Could you check a few things on this model? Use its own coordinates, in mm. Face numbers are marked on the shaded views. A direction names the side the tool comes from. Give positions to 0.01 mm unless a question says otherwise; leave off trailing zeros. Order: outer loops, then holes, each group sorted by start corner. A loop starts at its lowest first (then second) coordinate and runs counter-clockwise, first axis right, second up. Notation, with made-up numbers: (-3.75, -36) - (30.25, -36) arc R11 ccw to (30.25, -18) - close; hole circle Ø4 at (70.5, 18.25). An arc over 180 degrees is marked (long way). Put each result on its own line as item: value.
Autodesk Inventor part; units mm, degrees
ref_plane "YZ Plane" through (0, 0, 0) normal (1, 0, 0) x (0, 1, 0)
ref_plane "XZ Plane" through (0, 0, 0) normal (0, 1, 0) x (-1, 0, 0)
ref_plane "XY Plane" through (0, 0, 0) normal (0, 0, 1) x (1, 0, 0)
sketch "Sketch1" plane through (0, 0, 0) normal (0, 1, 0) x (-1, 0, 0)
  line L0 (-15, 15) -> (15, 15)
  line L1 (15, 15) -> (15, -15)
  line L2 (15, -15) -> (-15, -15)
  line L3 (-15, -15) -> (-15, 15)
  line L4 (-15, 15) -> (15, -15) construction
  line L5 (15, 15) -> (-15, -15) construction
  line L6 (-15, -15) -> (-15, -25)
  line L7 (-15, -25) -> (15, -15)
  point P0 (0, 0)
  dimension "d0" = 30
  dimension "d1" = 30
  dimension "d2" = 10
extrude "Extrusion1" add sketch "Sketch1" along normal blind 5
sketch "Sketch2" plane through (0, 5, 0) normal (0, 1, 0) x (1, 0, 0)
  line L0 (15, 25) -> (-15, 15)
  line L1 (15, 25) -> (18.0837, 15.7488)
  line L2 (15, -15) -> (15, 25)
  line L3 (15, 25) -> (6.9886, 22.3295)
  line L4 (-15, 15) -> (-9.6166, 16.7945)
  line L5 (-15, 15) -> (-13.1902, 9.5707)
  point P0 (0, 0)
ref_plane "Work Plane2" through (-15, 5, -15) normal (-0.9487, 0, 0.3162) x (0, -1, 0)
sketch "Sketch3" plane through (-15, 5, -15) normal (-0.9487, 0, 0.3162) x (0, -1, 0)
  line L0 (0, 37.9473) -> (0, 0)
  line L1 (0, 0) -> (-5, 0)
  line L2 (-5, 0) -> (-5, 3)
  line L3 (-3, 5) -> (0, 5)
  line L4 (0, 0) -> (0, 5)
  arc A0 (-3, 5) -> (-5, 3) centre (-3, 3) ccw
  line L5 (0, 0) -> (5.0254, 0) construction
  line L6 (5, 0) -> (0, 0)
  line L7 (0, 0) -> (-5, -1.8199)
  line L8 (0, 0) -> (5.3209, 0) construction
  line L9 (-5, -1.8199) -> (-5, 0)
  line L10 (0, 0) -> (-3.2889, -1.1971)
  line L11 (0, 0) -> (-2.8191, -1.0261)
  line L12 (0, 0) -> (1.5391, -4.2286)
  line L13 (1.5391, -4.2286) -> (-2.6895, -5.7677)
  line L14 (-2.6895, -5.7677) -> (-2.8191, -1.0261)
  point P0 (5, 18.9737)
  point P1 (-5, 5)
  dimension "d5" = 5
  dimension "d6" = 5
  dimension "d7" = 2
  dimension "d9" = 160
  dimension "d12" = 3.5
  dimension "d20" = 3
  dimension "d21" = 4.5
extrude "Extrusion2" add sketch "Sketch3" against normal blind 30
ref_plane "Work Plane4" through (-16.8239, 7.6895, -20.4717) normal (0.1082, -0.9397, 0.3245) x (0.9487, 0, -0.3162)
sketch "Sketch5" plane through (-16.8239, 7.6895, -20.4717) normal (0.1082, -0.9397, 0.3245) x (0.9487, 0, -0.3162)
  line L0 (30, 4.5) -> (30, 0)
  line L1 (30, 0) -> (30, -0.5)
  line L2 (30, -0.5) -> (15, -0.5)
  line L3 (15, -0.5) -> (15, 2)
  circle A0 centre (15, 2) radius 1.5
  point P0 (9.4868, 20.6193)
  dimension "d24" = 0.5
  dimension "d25" = 15
  dimension "d26" = 2.5
  dimension "d27" = 3
extrude "Extrusion4" cut sketch "Sketch5" along normal blind 10
sketch "Sketch6" plane through (0, 5, 0) normal (0, 1, 0) x (1, 0, 0)
  circle A0 centre (0, 0) radius 6.75
  line L0 (-6.75, 3.8971) -> (0, 7.7942)
  line L1 (0, 7.7942) -> (6.75, 3.8971)
  line L2 (6.75, 3.8971) -> (6.75, -3.8971)
  line L3 (6.75, -3.8971) -> (0, -7.7942)
  line L4 (0, -7.7942) -> (-6.75, -3.8971)
  line L5 (-6.75, -3.8971) -> (-6.75, 3.8971)
  circle A1 centre (0, 0) radius 3.5
  point P0 (-6.75, 0)
  dimension "d43" = 13.5
  dimension "d44" = 7
extrude "Extrusion5" add sketch "Sketch6" along normal blind 4.25
sketch "Sketch7" plane through (-15, 5, -15) normal (-0.9487, 0, 0.3162) x (0, -1, 0)
  line L0 (0, 0) -> (6.5506, 2.3842)
  line L1 (0, 0) -> (6.971, 0) construction
  line L2 (6.5506, 2.3842) -> (6.5506, -3.325)
  line L3 (6.5506, -3.325) -> (0, 0)
  point P0 (5, 18.9737)
  dimension "d34" = 20
extrude "Extrusion6" cut sketch "Sketch7" along normal blind 5 and the other way blind 40
fillet "Fillet2" radius 0.5 1 edges at (-2.5937, 7.6895, -25.2151)
sketch "Sketch8" plane through (-13.4189, 5, -10.2566) normal (0.3162, 0, 0.9487) x (0.9487, 0, -0.3162)
  line L0 (30, 0) -> (31.6228, 0)
  line L1 (30, 0) -> (36.1043, 0)
  line L2 (36.1043, 0) -> (36.1043, -10.0041)
  line L3 (36.1043, -10.0041) -> (30, -10.0041)
  line L4 (30, -10.0041) -> (30, 0)
  point P0 (9.4868, -5)
extrude "Extrusion7" cut sketch "Sketch8" along normal mid plane 20
fillet "Fillet3" radius 10 2 edges at (15, 2.5, 15) (-15, 2.5, 15)
properties part number "sem2_thumbmount"
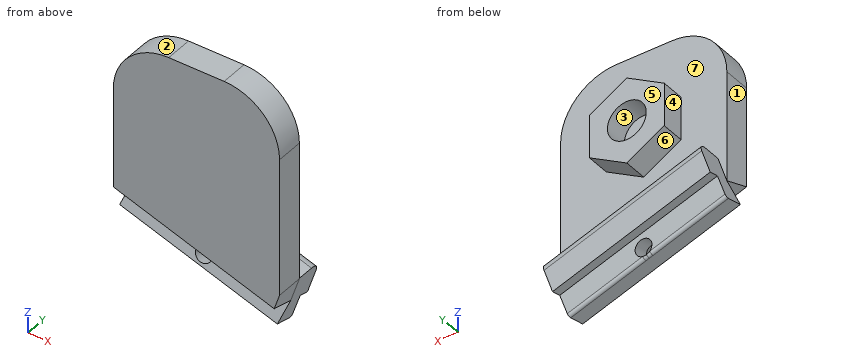
1) If I drill on line 1 (X direction, y = 8.45, z = 0); line 2 (Z direction, x = 0, y = 6.35); line 3 (Z direction, x = 0, y = 7), over which ranges is the centre line in solid material (lowest first)? Write a range as [from, to].
Filled in:
line 1: x = [-6.75, -3.5], [3.5, 6.75]
line 2: z = [-25.57, -14.73], [-7.79, -3.5], [3.5, 7.79]
line 3: z = [-25.81, -14.73], [-7.79, -3.5], [3.5, 7.79]
2) Which directions (+Z, -Z, +X, -X, +Y, -Y) give clear straight access to the entire face, cutting with the end or side of a thin tool? Please do the marked faces 4, 5, 6 and 7.
Filled in:
face 4: +Z, -X, +Y
face 5: +Z, +X, -X, +Y
face 6: -X, +Y
face 7: +Y
3) Suppose I cut it at A-A, the plane y = 5.75. State how many separate pieces and enclosed holes the cut face has, and give its area (3 significant figures).
Filled in:
separate pieces: 2
enclosed holes: 2
area: 414 mm^2
4) Suppose I cut it at D-D, the plane z = 7. List the corners of the cut face in (x, y) for me, and give its area (3 significant figures).
Filled in:
outline: (-14.8, 0) - (14.8, 0) - (14.8, 5) - (1.38, 5) - (1.38, 9.25) - (-1.38, 9.25) - (-1.38, 5) - (-14.8, 5) - close
area: 160 mm^2
5) Suppose I cut it at C-C, the plane y = 3. List the corners of the cut face in (x, z) for me.
Filled in:
outline: (-15, -14.23) - (13.69, -23.8) - (15, -19.87) - (15, 5) arc R10 ccw to (5, 15) - (-5, 15) arc R10 ccw to (-15, 5) - close
6) Suppose I cut it at B-B, the plane z = 0. List the corners of the cut face in (x, y) for me, and give its area (3 significant figures).
Filled in:
outline: (-15, 0) - (15, 0) - (15, 5) - (6.75, 5) - (6.75, 9.25) - (3.5, 9.25) - (3.5, 5) - (-3.5, 5) - (-3.5, 9.25) - (-6.75, 9.25) - (-6.75, 5) - (-15, 5) - close
area: 178 mm^2
7) We'd pull the mould along Z, two halves only. Please class the marked faces 1, 2 and 3: pulls with the +Z half, pulls with the -Z half, needs draft (parallel to the pull), parting line crosses it, or undercut.
Filled in:
face 1: needs draft
face 2: pulls with the +Z half
face 3: undercut
8) I'm going to push flat-ended pins straight in: pin 1 (3.5 mm diameter, centred on y = 6, z = 1.5, fed in from +X); pin 2 (2.5 mm diameter, centred on y = 2.5, z = -3, fed in from -X); pin 3 (4 mm diameter, centred on x = 1.5, z = 3, fed in from +Y). Where does each tip first touch, or does it pass through?
Filled in:
pin 1: stops at x = 15
pin 2: stops at x = -15
pin 3: stops at y = 9.25
